The model under review builds one solid part; all positions refer to its coordinate system, in mm. Round coordinates to 2 decimals unless told otherwise and drop trailing zeros. Loops run counter-clockwise (first coordinate to the right, second up) from the corner with the lowest first, then second, coordinate; pieces in that order, holes last. Notation, with made-up numbers: M -5.5,57.25 L 50.5,57.25 A29 ccw 50.5,90.25 Z; hole C 80.5,46 d8. An arc over 180 degrees is marked long. Return JSON: item names as keys, results as strings. Group by question number.
Q1. Consider section D-D (x = 0). State the section outline as (y, z) points (1 decimal).
Q2. Consider section C-C (x = -2.5). State the section outline as (y, z) points, and give its area (3 significant figures).
Q3. Consider section B-B (z = 0.25). Count the separate pieces of the cut face and the enclosed holes in it, and give its area (3 significant figures).
Q4. To check wall thickness, follow line 1 along Y through (x, z) = (0, 0.35) (1 decimal); line 2 along X through (y, z) = (0.5, 0.15); line 3 along Y through (x, z) = (1, 0.1). State the ranges of each line that lie inside material, in increasing order.
Q5. Draft analysis for pull direction Y (two halves, no side actions). For faces 1 (the face through (2.2, -2.5, 0.5)), 2 (the face through (0.141, 3.617, 0.246)), 3 (the face through (0.133, 3.172, 0.246)), state which applies: pulls with the +Y half, pulls with the -Y half, needs draft (parallel to the pull), parting line crosses it, or undercut.
Q6. Consider section A-A (y = 0). State the section outline as (x, z) points (1 decimal).
from build123d import *

# Parameters (mm, degrees)
SKETCH1_R           = 3.6195
SKETCH1_R_2         = 3.175
BOSS_EXTRUDE1_DEPTH = 0.5
CUT_EXTRUDE1_DEPTH  = 6.143108058
SKETCH3_W           = 0.762
SKETCH3_H           = 1.27
SKETCH3_R           = 0.1905
BOSS_EXTRUDE2_DEPTH = 0.5
FILLET1_R           = 0.254


with BuildPart() as part:
    # Sketch1 → Boss-Extrude1 (new body)
    with BuildSketch(Plane.XY):
        Circle(SKETCH1_R)
        Circle(SKETCH1_R_2, mode=Mode.SUBTRACT)
    extrude(amount=BOSS_EXTRUDE1_DEPTH)

    # Sketch2 → Cut-Extrude1 (cut, through all)
    with BuildSketch(Plane.XY.offset(0.5)):
        Polygon((0.5, -2.208183393), (0.5, -4.13884283), (-0.5, -4.13884283), (-0.5, -2.208183393), (-0.5, 2.208183393), (0.5, 2.208183393), align=None)
    extrude(amount=-CUT_EXTRUDE1_DEPTH, mode=Mode.SUBTRACT)

    # Sketch3 → Boss-Extrude2 (add)
    # profile 1 of 2: a face of its own
    with BuildSketch(Plane(origin=(0, 0, 0), x_dir=(-1, 0, 0), z_dir=(0, 0, -1))):
        with Locations((0.881, -3.770382752)):
            Rectangle(SKETCH3_W, SKETCH3_H)
        with Locations((0.881, -4.024382752)):
            Circle(SKETCH3_R, mode=Mode.SUBTRACT)
    # profile 2 of 2: a face of its own
    with BuildSketch(Plane(origin=(0, 0, 0), x_dir=(-1, 0, 0), z_dir=(0, 0, -1))):
        with Locations((-0.881, -3.770382752)):
            Rectangle(SKETCH3_W, SKETCH3_H)
        with Locations((-0.881, -4.024382752)):
            Circle(SKETCH3_R, mode=Mode.SUBTRACT)
    extrude(amount=-BOSS_EXTRUDE2_DEPTH)

    # Fillet1
    fillet1_edges = [part.edges().sort_by_distance(p)[0] for p in [
        (-0.5, -4.405382752, 0.25),
        (-1.262, -4.405382752, 0.25),
        (1.262, -4.405382752, 0.25),
        (0.5, -4.405382752, 0.25),
    ]]
    fillet(fillet1_edges, radius=FILLET1_R)


solid = part.part
Values:
{
 "1": {"outline": "M 3.2,0 L 3.6,0 L 3.6,0.5 L 3.2,0.5 Z"},
 "2": {"outline": "M -2.62,0 L -1.96,0 L -1.96,0.5 L -2.62,0.5 Z; M 1.96,0 L 2.62,0 L 2.62,0.5 L 1.96,0.5 Z", "area": "0.660 mm2"},
 "3": {"separate pieces": "1", "enclosed holes": "2", "area": "10.1 mm2"},
 "4": {"line 1": "y = 3.2 to 3.6", "line 2": "x = -3.58 to -3.14, 3.14 to 3.58", "line 3": "y = -4.41 to -4.17, -3.88 to -3.01, 3.01 to 3.48"},
 "5": {"face 1": "needs draft", "face 2": "parting line crosses it", "face 3": "undercut"},
 "6": {"outline": "M -3.6,0 L -3.2,0 L -3.2,0.5 L -3.6,0.5 Z; M 3.2,0 L 3.6,0 L 3.6,0.5 L 3.2,0.5 Z"}
}
